Source: three-view drawing plus pictorial views. Frame: mm from the lowest corner of the part. A direction names the side the tool comes from. Coordinates: 2 decimals unless noted, no trailing zeros. Write each loop counter-clockwise with the first axis right and the second up, starting at its lowest first coordinate (ties: lowest second). Pieces come first, ordered by that corner, then holes. Notation, with made-up numbers: (28, -12) - (50, -12) arc R17 ccw to (50, 5) - close; hole circle Ø3 at (84, 29). An arc over 180 degrees is marked (long way). One line per item, written item: value.
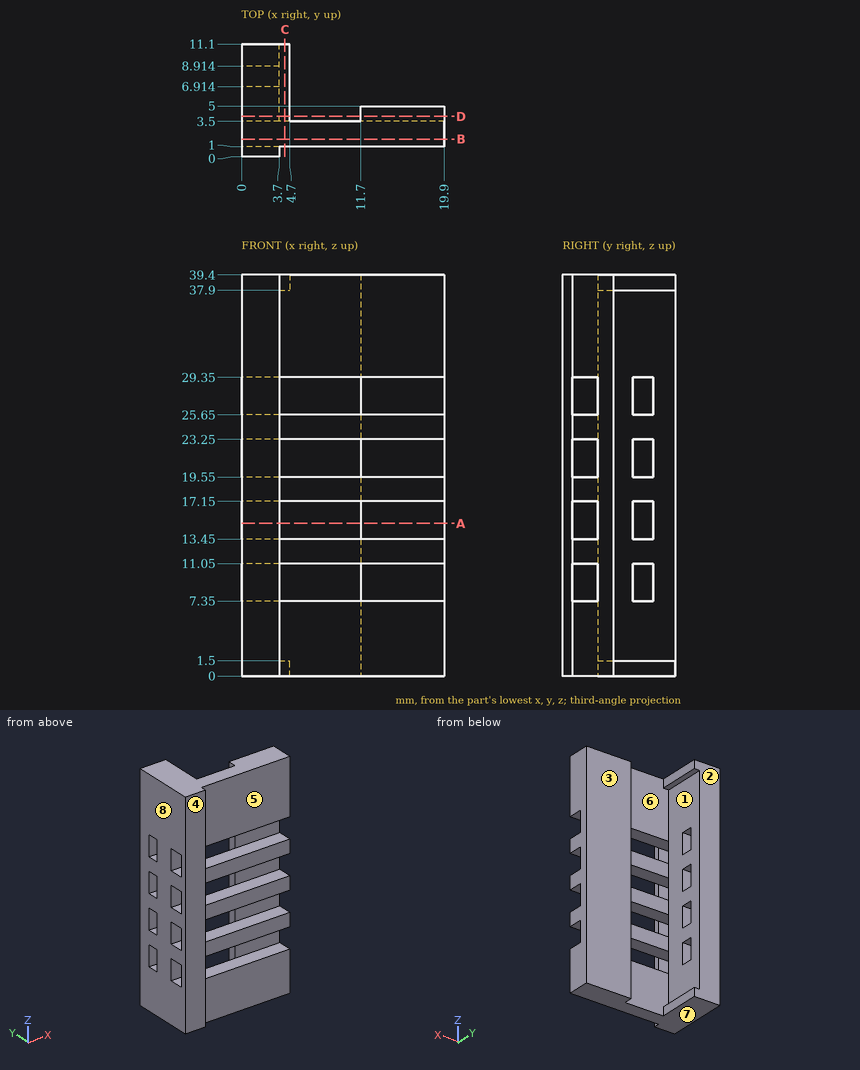
1) Draft query along X for the marked faces 6, 7 and 8. Return one class per face: released by +X, released by -X, zero draft, split by the parting line, or undercut.
Values found:
face 6: undercut
face 7: zero draft
face 8: released by -X
2) Section query C-C on x = 4.25. Output: boundary loops of the cut face in (y, z).
Values found:
outline: (1, 0) - (11.1, 0) - (11.1, 1.5) - (3.5, 1.5) - (3.5, 7.35) - (1, 7.35) - close; (1, 11.05) - (3.5, 11.05) - (3.5, 13.45) - (1, 13.45) - close; (1, 17.15) - (3.5, 17.15) - (3.5, 19.55) - (1, 19.55) - close; (1, 23.25) - (3.5, 23.25) - (3.5, 25.65) - (1, 25.65) - close; (1, 29.35) - (3.5, 29.35) - (3.5, 37.9) - (11.1, 37.9) - (11.1, 39.4) - (1, 39.4) - close
3) Material intervals for line 1 (Z direction, x = 7.5, y = 1.75); line 2 (Y direction, x = 12.5, z = 18.5), sorted ascending.
Values found:
line 1: 0 to 7.35, 11.05 to 13.45, 17.15 to 19.55, 23.25 to 25.65, 29.35 to 39.4
line 2: 1 to 5
4) Contact query for flat-ended pins moving along their axis: P1, Ø6, axis at y = 1.5, z = 35, coming from the -X side; P2, Ø1.5, axis at x = 9, y = 5, coming from the -Z side; P3, Ø3, axis at x = 6, z = 13, coming from the +Y side; P4, Ø1.9, axis at x = 15, z = 16, coming from the -Y side. Output: stop coordinate, or through.
Values found:
P1: x = 0
P2: through
P3: y = 3.5
P4: y = 3.5
5) Section query D-D on y = 4. Output: boundary loops of the cut face in (x, z).
Values found:
outline: (0, 0) - (4.7, 0) - (4.7, 1.5) - (3.7, 1.5) - (3.7, 37.9) - (4.7, 37.9) - (4.7, 39.4) - (0, 39.4) - close; (11.7, 0) - (19.9, 0) - (19.9, 39.4) - (11.7, 39.4) - close
6) Section query B-B on y = 1.75. Output: boundary loops of the cut face in (x, z).
Values found:
outline: (0, 0) - (19.9, 0) - (19.9, 7.35) - (0, 7.35) - close; (0, 11.05) - (19.9, 11.05) - (19.9, 13.45) - (0, 13.45) - close; (0, 17.15) - (19.9, 17.15) - (19.9, 19.55) - (0, 19.55) - close; (0, 23.25) - (19.9, 23.25) - (19.9, 25.65) - (0, 25.65) - close; (0, 29.35) - (19.9, 29.35) - (19.9, 39.4) - (0, 39.4) - close
7) Reachability of the marked faces 1, 2, 3, 4 and 5 from +Z, -Z, +X, -X, +Y, -Y: full face, straight path, thin tool, end or side. Return the list, or none.
Values found:
face 1: +Y
face 2: +Z, -Z, +X, -X, +Y
face 3: +Z, -Z, +X, +Y
face 4: +Z, -Z, +X, -X, -Y
face 5: +Z, -Z, +X, -Y
8) Section query A-A on z = 15. Output: boundary loops of the cut face in (x, y) (1 decimal).
Values found:
outline: (0, 0) - (3.7, 0) - (3.7, 1) - (0, 1) - close; (0, 3.5) - (3.7, 3.5) - (3.7, 6.9) - (0, 6.9) - close; (0, 8.9) - (3.7, 8.9) - (3.7, 11.1) - (0, 11.1) - close; (11.7, 3.5) - (19.9, 3.5) - (19.9, 5) - (11.7, 5) - close
